from build123d import *

# Parameters (mm, degrees)
FILLET1_R            = 10
SHELL1_T             = -3.175
SKETCH7_W            = 10
SKETCH7_H            = 39
SKETCH7_R            = 1
BOSS_EXTRUDE1_DEPTH  = 10
FILLET2_R            = 4
FILLET2_OF_MIRROR1_R = 4


with BuildPart() as part:
    # Sketch1 → Loft3 section 0
    with BuildSketch(Plane(origin=(0, 0, 0), x_dir=(1, 0, 0), z_dir=(0, 1, 0))):
        with BuildLine():
            Line((111.125, -92.075), (-111.125, -92.075))
            Line((-111.125, -92.075), (-111.125, 92.075))
            Line((-111.125, 92.075), (111.125, 92.075))
            Line((111.125, 92.075), (111.125, -92.075))
        make_face()
    # Sketch2 → Loft3 section 1
    with BuildSketch(Plane(origin=(0, 25.4, 0), x_dir=(1, 0, 0), z_dir=(0, 1, 0))):
        with BuildLine():
            Line((111.125, 92.075), (-111.125, 92.075))
            Line((-111.125, 92.075), (-111.125, -92.075))
            Line((-111.125, -92.075), (111.125, -92.075))
            Line((111.125, -92.075), (111.125, 92.075))
        make_face()
    loft()

    # Fillet1
    fillet1_edges = [part.edges().sort_by_distance(p)[0] for p in [
        (0, 25.4, -92.075),
        (111.125, 25.4, 0),
        (0, 25.4, 92.075),
        (-111.125, 25.4, 0),
        (111.125, 12.7, -92.075),
        (111.125, 12.7, 92.075),
        (-111.125, 12.7, -92.075),
        (-111.125, 12.7, 92.075),
    ]]
    fillet(fillet1_edges, radius=FILLET1_R)

    # Shell1
    shell1_openings = [part.faces().sort_by_distance(p)[0] for p in [
        (-6.8e-08, 0, 8.2e-08),
    ]]
    offset(amount=SHELL1_T, openings=shell1_openings)

    # Sketch7 → Boss-Extrude1 (add)
    with BuildSketch(Plane(origin=(70, 0, 0), x_dir=(0, 0, -1), z_dir=(1, 0, 0))):
        with Locations((97.075, -4.1)):
            Rectangle(SKETCH7_W, SKETCH7_H)
        with Locations((95.075, -18.2245)):
            Circle(SKETCH7_R, mode=Mode.SUBTRACT)
    boss_extrude1 = extrude(amount=BOSS_EXTRUDE1_DEPTH)

    # Fillet2
    fillet2_edges = [part.edges().sort_by_distance(p)[0] for p in [
        (75, -23.6, -102.075),
        (75, 15.4, -102.075),
        (70, -23.6, -97.075),
        (75, -23.6, -92.075),
        (80, -23.6, -97.075),
    ]]
    fillet(fillet2_edges, radius=FILLET2_R)

    # Mirror1: Boss-Extrude1 across plane
    add(boss_extrude1.mirror(Plane(origin=(0, 0, 0), x_dir=(0, 0, 1), z_dir=(1, 0, 0))))

    # Fillet2 of Mirror1
    fillet2_of_mirror1_edges = [part.edges().sort_by_distance(p)[0] for p in [
        (-75, -23.6, -102.075),
        (-75, 15.4, -102.075),
        (-70, -23.6, -97.075),
        (-75, -23.6, -92.075),
        (-80, -23.6, -97.075),
    ]]
    fillet(fillet2_of_mirror1_edges, radius=FILLET2_OF_MIRROR1_R)


solid = part.part
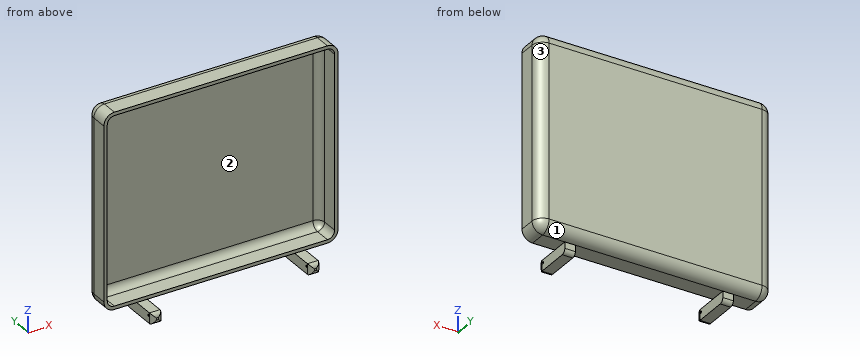
Geometry: final body of the model. Coordinates: model frame, mm. Face numbers are marked on the shaded views. Round coordinates to 2 decimals unless told otherwise and drop trailing zeros. Loops run counter-clockwise (first coordinate to the right, second up) from the corner with the lowest first, then second, coordinate; pieces in that order, holes last. Notation, with made-up numbers: M 30,10.25 L 63,10.25 A12 ccw 63,15.25 Z; hole C 72.5,83.25 d5. An arc over 180 degrees is marked long. One line per question, with ' | ' between items.
(1) Cut plane A-A on y = -4.5. Return the cut outline in (x, z) (3 decimals).
Check result:
outline: M -80,-102.075 L -70,-102.075 L -70,-92.075 L -80,-92.075 Z; M 70,-102.075 L 80,-102.075 L 80,-92.075 L 70,-92.075 Z
(2) Cut plane B-B on z = -49. Return the cut outline in (x, y) (3 decimals).
Check result:
outline: M -111.125,0 L -107.95,0 L -107.95,15.4 A6.825 cw -101.125,22.225 L 101.125,22.225 A6.825 cw 107.95,15.4 L 107.95,0 L 111.125,0 L 111.125,15.4 A10 ccw 101.125,25.4 L -101.125,25.4 A10 ccw -111.125,15.4 Z
(3) Cut plane D-D on y = 19. Return the cut outline in (x, z) (3 decimals).
Check result:
outline: M -110.455,-82.075 A9.33 ccw -101.125,-91.405 L 101.125,-91.405 A9.33 ccw 110.455,-82.075 L 110.455,82.075 A9.33 ccw 101.125,91.405 L -101.125,91.405 A9.33 ccw -110.455,82.075 Z; hole M -106.923,-82.075 A5.798 ccw -101.125,-87.873 L 101.125,-87.873 A5.798 ccw 106.923,-82.075 L 106.923,82.075 A5.798 ccw 101.125,87.873 L -101.125,87.873 A5.798 ccw -106.923,82.075 Z
(4) Contact query for flat-ended pins moving along their axis: P1, Ø5, axis at x = -83, y = -16, coming from the -Z side; P2, Ø11, axis at x = 77, y = -14, coming from the +Z side (3 decimals); P3, Ø8, axis at y = -6, z = -99.5, coming from the -X side; P4, Ø4.5, axis at x = 25.5, y = 5, coming from the -Z side (3 decimals). Output: stop coordinate, or through.
Check result:
P1: passes through | P2: stops at z = -92.075 | P3: stops at x = -80 | P4: stops at z = -92.075
(5) Cut plane C-C on x = -57. Return the cut outline in (y, z) (3 decimals), plus the area to 3 significant figures.
Check result:
outline: M 0,-92.075 L 15.4,-92.075 A10 ccw 25.4,-82.075 L 25.4,82.075 A10 ccw 15.4,92.075 L 0,92.075 L 0,88.9 L 15.4,88.9 A6.825 cw 22.225,82.075 L 22.225,-82.075 A6.825 cw 15.4,-88.9 L 0,-88.9 Z | area: 703 mm2
(6) Pull-direction query (X, two-part tool) for the marked faces 1, 2 and 3; classes: +X half, -X half, draft (parallel to the pull), parting line (faces both ways), or undercut.
Check result:
face 1: draft | face 2: undercut | face 3: +X half
(7) Material intervals for line 1 along X through (y, z) = (14.5, 30.5) (3 decimals); line 2 along Z through (x, y) = (-51.5, 16); line 3 along Z through (x, y) = (76.5, 1) (3 decimals), sorted ascending. Write a range as from..to.
Check result:
line 1: x = -111.125..-107.95, 107.95..111.125 | line 2: z = -92.06..-88.87, 88.87..92.06 | line 3: z = -102.075..-88.9, 88.9..92.075
